Design review of the part built by this model. Coordinates are the model's own, in mm. Coordinates: 2 decimals unless noted, no trailing zeros. Write each loop counter-clockwise with the first axis right and the second up, starting at its lowest first coordinate (ties: lowest second). Pieces come first, ordered by that corner, then holes. Notation, with made-up numbers: (-5, 61.5) - (7, 61.5) arc R21 cw to (7, 69.5) - close; hole circle Ø4 at (-20.5, 85.5). An arc over 180 degrees is marked (long way). One line per item, written item: value.
from build123d import *

# Parameters (mm, degrees)
F0_R     = 20
F0_R_2   = 2.032
F1_DEPTH = 50
F2_SIZE2 = 18.6602540378
F2_SIZE  = 5
F3_SIZE  = 15


with BuildPart() as f1:
    # F0 (on Front) → F1 (new body)
    with BuildSketch(Plane.XZ):
        Circle(F0_R)
        Circle(F0_R_2, mode=Mode.SUBTRACT)
    extrude(amount=F1_DEPTH)

    # F2
    f2_edges = [f1.edges().sort_by_distance(p)[0] for p in [
        (-20, -50, 0),
    ]]
    f2_side = f1.faces().sort_by_distance((-19.434315, -50, 0))[0]
    chamfer(f2_edges, length=F2_SIZE, length2=F2_SIZE2, reference=f2_side)

    # F3
    f3_edges = [f1.edges().sort_by_distance(p)[0] for p in [
        (-20, 0, 0),
    ]]
    chamfer(f3_edges, length=F3_SIZE)


solid = f1.part
1. Insertion check: pin 1 Ø3 at (x, z) = (-15, 14) entering from +Y; pin 2 Ø2 at (y, z) = (-35.5, 8.5) entering from -X; pin 3 Ø4 at (x, y) = (-9, -29) entering from -Z (3 decimals). Each pin has a flat end and moves straight along its axis. Give the tip position at first contact, or say it passes through.
Answer block:
pin 1: stops at y = -14.02
pin 2: stops at x = -17.42
pin 3: stops at z = -18.735
2. Consider section C-C, the plane y = -7. Write out the cut boundary in (x, z).
Answer block:
outline: circle Ø24 at (0, 0); hole circle Ø4.06 at (0, 0)
3. Consider section B-B, the plane x = 0. Write out the cut boundary in (y, z).
Answer block:
outline: (-50, -15) - (-31.34, -20) - (-15, -20) - (0, -5) - (0, -2.03) - (-50, -2.03) - close; (-50, 2.03) - (0, 2.03) - (0, 5) - (-15, 20) - (-31.34, 20) - (-50, 15) - close
4. Consider section A-A, the plane z = 0. Write out the cut boundary in (x, y), then the cut area to 3 significant figures.
Answer block:
outline: (-20, -31.34) - (-15, -50) - (-2.03, -50) - (-2.03, 0) - (-5, 0) - (-20, -15) - close; (2.03, -50) - (15, -50) - (20, -31.34) - (20, -15) - (5, 0) - (2.03, 0) - close
area: 1,480 mm^2
5. Wall thickness on line 1 along Z through (x, y) = (0, -16); line 2 along Z through (x, y) = (0, -13); line 3 along Z through (x, y) = (-10, -29): over which ranges is each line inside the solid? List them lowest first.
Answer block:
line 1: z = -20 to -2.03, 2.03 to 20
line 2: z = -18 to -2.03, 2.03 to 18
line 3: z = -17.32 to 17.32
6. Consider section D-D, the plane y = -16. Write out the cut boundary in (x, z), then the cut area to 3 significant figures.
Answer block:
outline: circle Ø40 at (0, 0); hole circle Ø4.06 at (0, 0)
area: 1,240 mm^2
7. Mouldability with a two-part tool opening along X and no side actions: class faces 1 (the face through (0, -50, -3)), 2 (the face through (-0.44, -24.65, -1.984)), 3 (the face through (-1.242, -0.728, -5.592)) as released by +X, released by -X, zero draft, split by the parting line, or undercut.
Answer block:
face 1: zero draft
face 2: undercut
face 3: split by the parting line
